Study the drawing (mm; zero at the part's minimum x, y, z) and answer. Round coordinates to 2 decimals unless told otherwise and drop trailing zeros. Loops run counter-clockwise (first coordinate to the right, second up) from the corner with the lowest first, then second, coordinate; pieces in that order, holes last. Notation, with made-up numbers: (-0.75, -3) - (50.25, -3) arc R9 ccw to (50.25, 10) - close; hole circle Ø4 at (45.25, 59). An arc over 180 degrees is marked (long way). Use CSV: the item, a comma, the result in double quotes. Start each with the question number.
1. Find section A-A (x = 5). Give the vertices of the cut face in (y, z).
2. Find section B-B (z = 5). Give the vertices of the cut face in (x, y), and give its area (3 significant figures).
3. Given pin 1 Ø4.5 at (x, z) = (195, 5) entering from -Y, flat-ended and moving along its own axis, determine where the tip first touches the part or whether it passes through.
4. Consider line 1 along X through (y, z) = (2.2, 115). Determine where the line is inside the solid, lowest interval first.
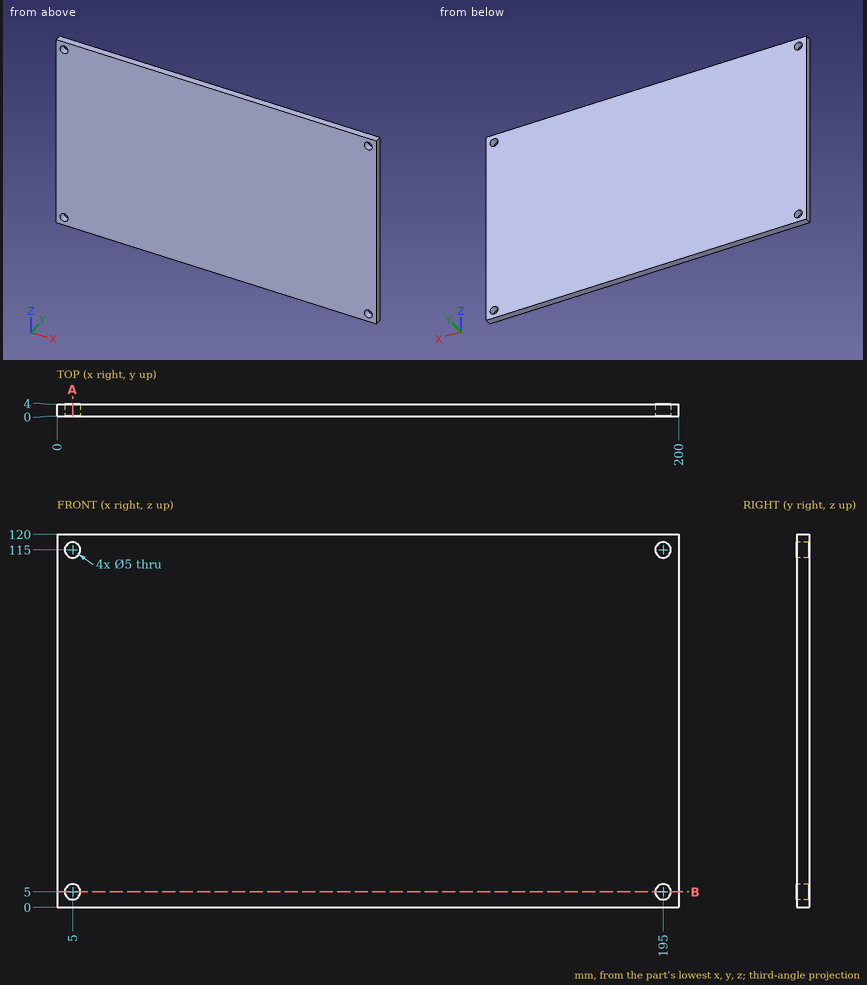
Filled sheet:
1,outline,"(0, 0) - (4, 0) - (4, 2.5) - (0, 2.5) - close; (0, 7.5) - (4, 7.5) - (4, 112.5) - (0, 112.5) - close; (0, 117.5) - (4, 117.5) - (4, 120) - (0, 120) - close"
2,outline,"(0, 0) - (2.5, 0) - (2.5, 4) - (0, 4) - close; (7.5, 0) - (192.5, 0) - (192.5, 4) - (7.5, 4) - close; (197.5, 0) - (200, 0) - (200, 4) - (197.5, 4) - close"
2,area,"760 mm²"
3,pin 1,"passes through"
4,line 1,"x = 0 to 2.5, 7.5 to 192.5, 197.5 to 200"
